Source: CAD feature listing. Evaluate the final solid. Frame: model axes, mm. Face numbers are marked on the shaded views. A direction names the side the tool comes from. Give positions to 0.01 mm unless a question says otherwise; leave off trailing zeros. Loops run counter-clockwise (first coordinate to the right, second up) from the corner with the lowest first, then second, coordinate; pieces in that order, holes last. Notation, with made-up numbers: M 57,49.5 L 89,49.5 A23 cw 89,79.5 Z; hole C -7,8.5 d1. An arc over 180 degrees is marked long. Answer in a Markdown table with one row per item.
```python
from build123d import *

# Parameters (mm, degrees)
F0_R     = 20
F1_DEPTH = 15
F2_R     = 18
F3_DEPTH = 13
F4_R     = 3.5
F4_R_2   = 1.5
F5_DEPTH = 13
F7_DEPTH = 100


with BuildPart() as f1:
    # F0 (on Top) → F1 (new body)
    with BuildSketch(Plane.XY):
        Circle(F0_R)
    extrude(amount=F1_DEPTH)

    # F2 (on face) → F3 (cut)
    with BuildSketch(Plane.XY.offset(15)):
        Circle(F2_R)
    extrude(amount=-F3_DEPTH, mode=Mode.SUBTRACT)

    # F4 (on face) → F5 (join)
    with BuildSketch(Plane.XY.offset(2)):
        Circle(F4_R)
        Circle(F4_R_2, mode=Mode.SUBTRACT)
    extrude(amount=F5_DEPTH)

    # F6 (on face) → F7 (cut)
    with BuildSketch(Plane.XY.offset(2)):
        with BuildLine():
            Line((-9.4231661407, -15.3363600598), (-3.0310889132, -1.75))
            Line((-3.0310889132, -1.75), (-17.9932604837, -0.4925212321))
            ThreePointArc((-17.9932604837, -0.4925212321), (-15.5884572681, -9), (-9.4231661407, -15.3363600598))
        make_face()
        with BuildLine():
            Line((-8.570094343, 15.8288812919), (0, 3.5))
            Line((0, 3.5), (8.570094343, 15.8288812919))
            ThreePointArc((8.570094343, 15.8288812919), (0, 18), (-8.570094343, 15.8288812919))
        make_face()
        with BuildLine():
            Line((17.9932604837, -0.4925212321), (3.0310889132, -1.75))
            Line((3.0310889132, -1.75), (9.4231661407, -15.3363600598))
            ThreePointArc((9.4231661407, -15.3363600598), (15.5884572681, -9), (17.9932604837, -0.4925212321))
        make_face()
    extrude(amount=-F7_DEPTH, mode=Mode.SUBTRACT)


solid = f1.part
```
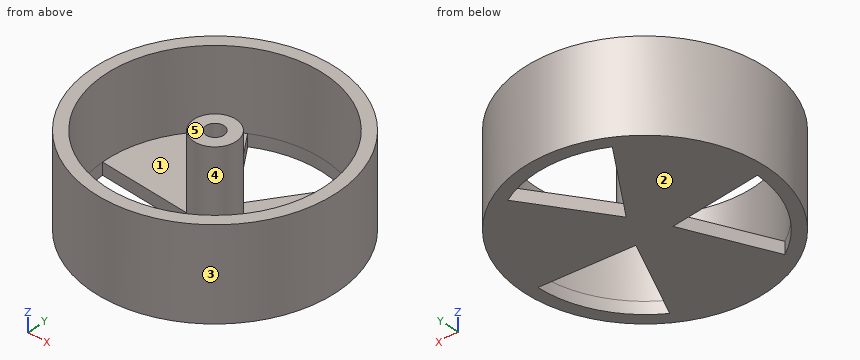
Q1. Section query C-C (z = 13.5). Output: boundary loops of the cut face in (x, y).
Values follow:
| item | result |
|---|---|
| outline | C 0,0 d40; C 0,0 d7; hole C 0,0 d36; hole C 0,0 d3 |
Q2. Section query D-D (y = -9). Output: boundary loops of the cut face in (x, z).
Values follow:
| item | result |
|---|---|
| outline | M -17.86,0 L -15.59,0 L -15.59,15 L -17.86,15 Z; M -6.44,0 L 6.44,0 L 6.44,2 L -6.44,2 Z; M 15.59,0 L 17.86,0 L 17.86,15 L 15.59,15 Z |
Q3. Ray query, probe 1 along Y at (x, z) = (0, 6.25); probe 2 along X at (y, z) = (3, 8.75); probe 3 along X at (y, z) = (0.5, 2.25). Return the intervals inside material, ascending. Write a range as from..to.
Values follow:
| item | result |
|---|---|
| probe 1 | -20..-18, -3.5..-1.5, 1.5..3.5, 18..20 |
| probe 2 | -19.77..-17.75, -1.8..1.8, 17.75..19.77 |
| probe 3 | -19.99..-17.99, -3.46..-1.41, 1.41..3.46, 17.99..19.99 |
Q4. Section query A-A (y = 15). Output: boundary loops of the cut face in (x, z).
Values follow:
| item | result |
|---|---|
| outline | M -13.23,0 L -7.99,0 L -7.99,2 L -9.95,2 L -9.95,15 L -13.23,15 Z; M 7.99,0 L 13.23,0 L 13.23,15 L 9.95,15 L 9.95,2 L 7.99,2 Z |
Q5. Contact query for flat-ended pins moving along their axis: pin 1 Ø4 at (y, z) = (7, 6) entering from +X; pin 2 Ø2.5 at (x, y) = (0, 0) entering from +Z; pin 3 Ø1 at (x, z) = (14, 11) entering from -Y; pin 4 Ø18 at (x, y) = (2.5, -9.5) entering from +Z. Output: stop coordinate, or through.
Values follow:
| item | result |
|---|---|
| pin 1 | x = 19.36 |
| pin 2 | z = 2 |
| pin 3 | y = -14.76 |
| pin 4 | z = 15 |
Q6. Section query B-B (x = 14). Output: boundary loops of the cut face in (y, z), plus the area to 3 significant figures.
Values follow:
| item | result |
|---|---|
| outline | M -14.28,0 L -11.31,0 L -11.31,15 L -14.28,15 Z; M -0.83,0 L 14.28,0 L 14.28,15 L 11.31,15 L 11.31,2 L -0.83,2 Z |
| area | 113 mm^2 |
Q7. Mould query, pull axis Y, two halves, no side actions, for the marked faces 1, 2 and 3. Classes: +Y half, -Y half, draft (parallel to the pull), parting line (faces both ways), or undercut.
Values follow:
| item | result |
|---|---|
| face 1 | undercut |
| face 2 | draft |
| face 3 | parting line |
Q8. Reachability of the marked faces 4 and 5 from +Z, -Z, +X, -X, +Y, -Y: full face, straight path, thin tool, end or side. Return the list, or none.
Values follow:
| item | result |
|---|---|
| face 4 | +Z |
| face 5 | +Z, +X, -X, +Y, -Y |
